from build123d import *

# Parameters (mm, degrees)
SKETCH1_W             = 19.05
SKETCH1_H             = 9.525
BOSS_EXTRUDE1_DEPTH   = 79.375
SKETCH2_W             = 19.05
SKETCH2_H             = 25.4
CUT_EXTRUDE1_DEPTH    = 4.7625
M3_CLEARANCE_HOLE1_D  = 3.4
SKETCH5_R             = 5.55625
CUT_EXTRUDE2_DEPTH    = 3.96875
F_8_CLEARANCE_HOLE1_D = 4.4958
FILLET1_R             = 6.35


with BuildPart() as part:
    # Sketch1 → Boss-Extrude1 (new, symmetric)
    with BuildSketch(Plane.XY):
        Rectangle(SKETCH1_W, SKETCH1_H)
    extrude(amount=BOSS_EXTRUDE1_DEPTH, both=True)

    # Sketch2 → Cut-Extrude1 (cut)
    with BuildSketch(Plane(origin=(0, 4.7625, 0), x_dir=(1, 0, 0), z_dir=(0, 1, 0))):
        Rectangle(SKETCH2_W, SKETCH2_H)
    extrude(amount=-CUT_EXTRUDE1_DEPTH, mode=Mode.SUBTRACT)

    # M3 Clearance Hole1 (through all)
    with Locations(Plane(origin=(0, 4.7625, 0), x_dir=(1, 0, 0), z_dir=(0, 1, 0))):
        with Locations((0, -60.000000015), (0, 60.000000015)):
            Hole(M3_CLEARANCE_HOLE1_D / 2)

    # Sketch5 → Cut-Extrude2 (cut)
    with BuildSketch(Plane(origin=(0, 4.7625, 0), x_dir=(1, 0, 0), z_dir=(0, 1, 0))):
        with Locations(Location((0, -60.000000015, 0), (0, 0, 270))):
            Circle(SKETCH5_R)
        with Locations(Location((0, 60.000000015, 0), (0, 0, 270))):
            Circle(SKETCH5_R)
    extrude(amount=-CUT_EXTRUDE2_DEPTH, mode=Mode.SUBTRACT)

    # #8 Clearance Hole1 (through all)
    with Locations(Plane(origin=(0, 4.7625, 0), x_dir=(1, 0, 0), z_dir=(0, 1, 0))):
        with Locations((0, -73.025), (0, 73.025)):
            Hole(F_8_CLEARANCE_HOLE1_D / 2)

    # Fillet1
    fillet1_edges = [part.edges().sort_by_distance(p)[0] for p in [
        (-9.525, 0, 79.375),
        (9.525, 0, 79.375),
        (-9.525, 0, -79.375),
        (9.525, 0, -79.375),
    ]]
    fillet(fillet1_edges, radius=FILLET1_R)


solid = part.part
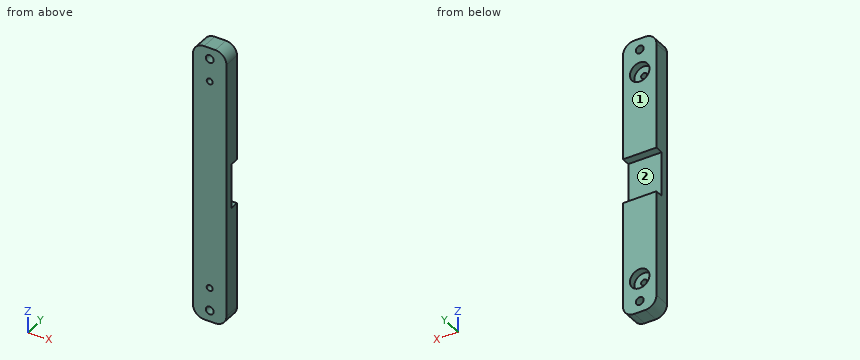
For this review, take the finished solid that the model builds, in its own axes (mm). Face numbers are marked on the shaded views. Round coordinates to 2 decimals unless told otherwise and drop trailing zeros. Loops run counter-clockwise (first coordinate to the right, second up) from the corner with the lowest first, then second, coordinate; pieces in that order, holes last. Notation, with made-up numbers: (-33.75, 65.5) - (-28.75, 65.5) arc R28 ccw to (-28.75, 96.5) - close; hole circle Ø1 at (34, -19.5). An arc over 180 degrees is marked (long way). One line per item, written item: value. Start each with the question number.
Item 1: Take a section at D-D (z = -10). Give the boundary of the cut face in (x, y) (1 decimal).
Item 2: For L1, parallel to Z at x = 0, y = -1.35 (3 decimals); L2, parallel to Z at x = 0.25, y = 3.75 (3 decimals); L3, parallel to X at y = 1.75, z = 60 (3 decimals), list the stretches that pass through material, from the lowest coordinate up.
Item 3: Clearance check with flat-ended pins moving along their axes: pin 1 Ø4 at (x, z) = (0, -73.025) entering from +Y; pin 2 Ø1.4 at (x, y) = (-4.5, 1.5) entering from +Z; pin 3 Ø4.5 at (x, z) = (0, -60) entering from +Y; pin 4 Ø5.5 at (x, z) = (3.5, 1.5) entering from +Y. State where each tip first meets the part, or that it passes through.
Item 4: The part is to be moulded in two halves that separate along Z. For the marked faces 1 and 2, say which applies: +Z half, -Z half, draft (parallel to the pull), parting line (faces both ways), or undercut.
Item 5: Take a section at A-A (y = 2.75). State how many separate pieces and enclosed holes the cut face has, plus the area to 3 significant figures.
Item 6: Take a section at B-B (z = -60). Give the boundary of the cut face in (x, y) (1 decimal), plus the area to 3 significant figures.
Answer below:
1. outline: (-9.5, -4.8) - (9.5, -4.8) - (9.5, 0) - (-9.5, 0) - close
2. L1: z = -79.375 to -75.273, -70.777 to -61.7, -58.3 to 58.3, 61.7 to 70.777, 75.273 to 79.375
2. L2: z = -79.375 to -75.259, -70.791 to -65.551, -54.449 to -12.7, 12.7 to 54.449, 65.551 to 70.791, 75.259 to 79.375
2. L3: x = -9.525 to -5.556, 5.556 to 9.525
3. pin 1: passes through
3. pin 2: stops at z = 79.34
3. pin 3: stops at y = 0.79
3. pin 4: stops at y = 0
4. face 1: draft
4. face 2: undercut
5. separate pieces: 2
5. enclosed holes: 4
5. area: 2,280 mm2
6. outline: (-9.5, -4.8) - (-1.7, -4.8) - (-1.7, 0.8) - (-5.6, 0.8) - (-5.6, 4.8) - (-9.5, 4.8) - close; (1.7, -4.8) - (9.5, -4.8) - (9.5, 4.8) - (5.6, 4.8) - (5.6, 0.8) - (1.7, 0.8) - close
6. area: 118 mm2
